Part model, mm, in its own coordinate system. Face numbers are marked on the shaded views. A direction names the side the tool comes from. Round coordinates to 2 decimals unless told otherwise and drop trailing zeros. Loops run counter-clockwise (first coordinate to the right, second up) from the corner with the lowest first, then second, coordinate; pieces in that order, holes last. Notation, with made-up numbers: (-15.5, 20) -> (43.5, 20) arc R13 ccw to (43.5, 45) -> close; hole circle Ø1 at (-21.5, 55). An arc over 180 degrees is marked (long way). Answer as CSV lines item,"result".
from build123d import *

# Parameters (mm, degrees)
F1_DEPTH = 40
F3_DEPTH = 35


with BuildPart() as f1:
    # F0 (on Top) → F1 (new body)
    with BuildSketch(Plane.XY):
        with BuildLine():
            Line((73.507474, 79.266992), (-73.638234, 79.266992))
            ThreePointArc((-73.638234, 79.266992), (-77.353579, 77.728046), (-78.892526, 74.0127))
            Line((-78.892526, 74.0127), (-78.892526, -73.133008))
            ThreePointArc((-78.892526, -73.133008), (-77.353579, -76.848354), (-73.638234, -78.3873))
            Line((-73.638234, -78.3873), (73.507474, -78.3873))
            ThreePointArc((73.507474, -78.3873), (77.22282, -76.848354), (78.761766, -73.133008))
            Line((78.761766, -73.133008), (78.761766, 74.0127))
            ThreePointArc((78.761766, 74.0127), (77.22282, 77.728046), (73.507474, 79.266992))
        make_face()
    extrude(amount=F1_DEPTH)

    # F2 (on face) → F3 (cut)
    with BuildSketch(Plane(origin=(0, 0, 0), x_dir=(1, 0, 0), z_dir=(0, 0, -1))):
        with BuildLine():
            Line((68.427474, 73.133008), (-68.558234, 73.133008))
            ThreePointArc((-68.558234, 73.133008), (-72.150336, 71.64511), (-73.638234, 68.053008))
            Line((-73.638234, 68.053008), (-73.638234, -68.9327))
            ThreePointArc((-73.638234, -68.9327), (-72.150336, -72.524802), (-68.558234, -74.0127))
            Line((-68.558234, -74.0127), (68.427474, -74.0127))
            ThreePointArc((68.427474, -74.0127), (72.019576, -72.524802), (73.507474, -68.9327))
            Line((73.507474, -68.9327), (73.507474, 68.053008))
            ThreePointArc((73.507474, 68.053008), (72.019576, 71.64511), (68.427474, 73.133008))
        make_face()
    extrude(amount=-F3_DEPTH, mode=Mode.SUBTRACT)


solid = f1.part
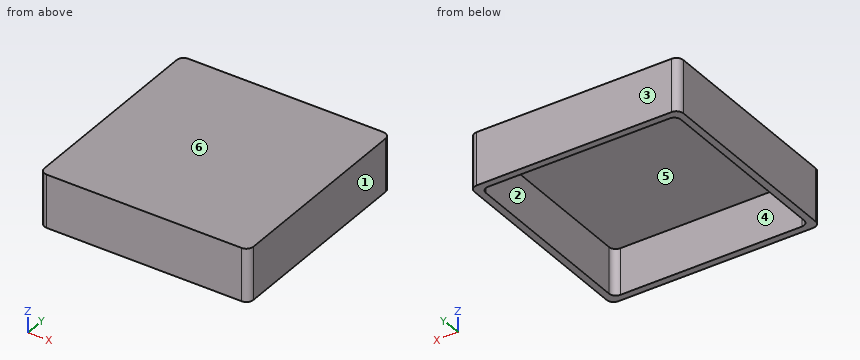
Q1. Saw through at A-A, the plane z = 11. Write the cut outline in (x, y), then the cut area to 3 significant figures.
Geometry results:
outline,"(-78.89, -73.13) arc R5.25 ccw to (-73.64, -78.39) -> (73.51, -78.39) arc R5.25 ccw to (78.76, -73.13) -> (78.76, 74.01) arc R5.25 ccw to (73.51, 79.27) -> (-73.64, 79.27) arc R5.25 ccw to (-78.89, 74.01) -> close; hole (-73.64, -68.05) arc R5.08 ccw to (-68.56, -73.13) -> (68.43, -73.13) arc R5.08 ccw to (73.51, -68.05) -> (73.51, 68.93) arc R5.08 ccw to (68.43, 74.01) -> (-68.56, 74.01) arc R5.08 ccw to (-73.64, 68.93) -> close"
area,"3,200 mm2"
Q2. Which spindle directions (+Z, -Z, +X, -X, +Y, -Y) get a long thin tool onto all of the face, cutting with end or side? Do the marked faces 1 and 2. Say none if no direction does.
Geometry results:
face 1,"+Z, -Z, +X, +Y, -Y"
face 2,"-Z"
Q3. Two-plate mould, pull along Y, no slides. Class the marked faces 3, 4, 5 and 6: pulls with the +Y half, pulls with the -Y half, needs draft (parallel to the pull), parting line crosses it, or undercut.
Geometry results:
face 3,"pulls with the +Y half"
face 4,"undercut"
face 5,"undercut"
face 6,"needs draft"
Q4. Saw through at B-B, the plane y = 14. Write the cut outline in (x, z).
Geometry results:
outline,"(-78.89, 0) -> (-73.64, 0) -> (-73.64, 35) -> (73.51, 35) -> (73.51, 0) -> (78.76, 0) -> (78.76, 40) -> (-78.89, 40) -> close"
Q5. Drill centre lines: line 1 along Y through (x, z) = (-13, 34.5); line 2 along X through (y, z) = (-37, 9); line 3 along Z through (x, y) = (-7, -25.5). Where is each one in solid material? Low to high.
Geometry results:
line 1,"-78.39 to -73.13, 74.01 to 79.27"
line 2,"-78.89 to -73.64, 73.51 to 78.76"
line 3,"35 to 40"
Q6. Saw through at C-C, the plane x = 16. Write the cut outline in (y, z), then the cut area to 3 significant figures.
Geometry results:
outline,"(-78.39, 0) -> (-73.13, 0) -> (-73.13, 35) -> (74.01, 35) -> (74.01, 0) -> (79.27, 0) -> (79.27, 40) -> (-78.39, 40) -> close"
area,"1,160 mm2"
Q7. Drop a flat-ended pin along its axis: P1, Ø12, axis at x = 35.5, y = -37.5, coming from the -Z side. Give the stop position or say it passes through.
Geometry results:
P1,"z = 35"
